Here's how the part is built. I have some questions about the finished solid (model axes, mm). Face numbers are marked on the shaded views. A direction names the side the tool comes from. Round coordinates to 2 decimals unless told otherwise and drop trailing zeros. Write each loop counter-clockwise with the first axis right and the second up, starting at its lowest first coordinate (ties: lowest second). Pieces come first, ordered by that corner, then holes. Notation, with made-up numbers: M -33,-27 L 19,-27 A12 ccw 19,-13 Z; hole C -21,-21 d11. An arc over 180 degrees is marked long. Write item = value, one per line. Start each with the question number.
(1) If we mould it in two halves opening along Y, with no side actions, what happens to the marked faces 6, 7 and 8? For each: released by +Y, released by -Y, zero draft, split by the parting line, or undercut.
(2) On a 3-axis mill with a long thin cutter (end or side, diameter ignored), from which of +Z, -Z, +X, -X, +Y, -Y can I reach the whole of each face in a straight line? I mean the marked faces 1, 2, 3, 4 and 5. Say none if no direction works.
(3) I want a section at A-A (y = 6.5). List the corners of the cut face in (x, z) for me.
(4) I want a section at C-C (y = -2.5). List the corners of the cut face in (x, z) for me, and give its area (3 significant figures).
(5) I want a section at D-D (x = 18.5). List the corners of the cut face in (y, z) for me, and give its area (3 significant figures).
(6) I want a section at B-B (z = -0.25). List the corners of the cut face in (x, y) for me, and give its area (3 significant figures).
(7) Will these pins go through, and if not, where does the flat tip stop? pin 1 Ø2 at (x, y) = (43, 12) entering from -Z; pin 2 Ø1 at (x, y) = (45.5, 10.5) entering from +Z; pin 3 Ø11 at (x, z) = (38, 1.5) entering from -Y.
(8) I need wall thicknesses on line 1 along X through (y, z) = (-0.5, 3.25); line 2 along Y through (x, z) = (6, 8.5); line 3 along X through (y, z) = (-3.25, 7.5). Which ranges of each line are inside material? Lowest first, please.
```python
from build123d import *

# Parameters (mm, degrees)
F1_DEPTH      = 5
F3_DEPTH      = 5
F3_DEPTH_BACK = 5


# Not quite as in the source:
# - a feature names something its author has since deleted; it is built from what else it names


with BuildPart() as f1:
    # F0 (on Front) → F1 (new body)
    with BuildSketch(Plane.XZ):
        Polygon((0, 9.7736853705), (0, 0), (0, -10.2263146295), (15, -10.2263146295), (15, 9.7736853705), align=None)
    extrude(amount=F1_DEPTH)

    # F2 (on Top) → F3 (join, two sides)
    with BuildSketch(Plane.XY) as f3_sk:
        Polygon((7.0152175973, 15), (7.0152175973, 0), (9.8953448171, 0), (9.8953448171, 10), (57.0152175973, 10), (57.0152175973, -4.3088319683), (60.7257795132, -4.3088319683), (60.7257795132, 15), align=None)
    extrude(amount=F3_DEPTH)
    extrude(f3_sk.sketch, amount=-F3_DEPTH_BACK)


solid = f1.part
```
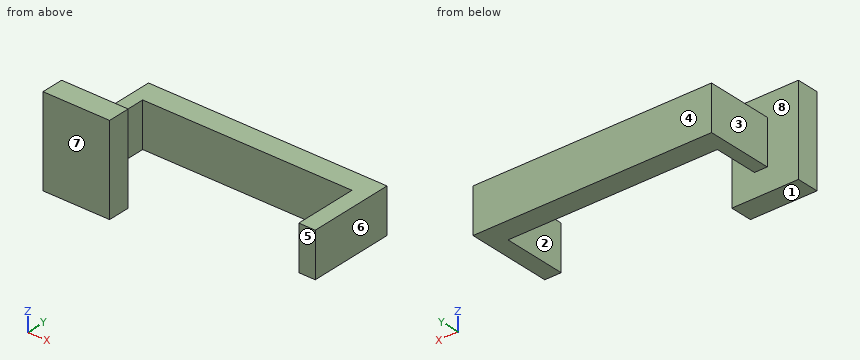
Returned:
q1.face_6 = zero draft
q1.face_7 = released by -Y
q1.face_8 = undercut
q2.face_1 = -Z, +X, -X, +Y, -Y
q2.face_2 = +Z, -Z, -Y
q2.face_3 = +Z, -Z, -X, +Y
q2.face_4 = +Z, -Z, +X, -X, +Y
q2.face_5 = +Z, -Z, +X, -Y
q3.outline = M 7.02,-5 L 9.9,-5 L 9.9,5 L 7.02,5 Z; M 57.02,-5 L 60.73,-5 L 60.73,5 L 57.02,5 Z
q4.outline = M 0,-10.23 L 15,-10.23 L 15,9.77 L 0,9.77 Z; M 57.02,-5 L 60.73,-5 L 60.73,5 L 57.02,5 Z
q4.area = 337 mm²
q5.outline = M 10,-5 L 15,-5 L 15,5 L 10,5 Z
q5.area = 50.0 mm²
q6.outline = M 0,-5 L 15,-5 L 15,0 L 9.9,0 L 9.9,10 L 57.02,10 L 57.02,-4.31 L 60.73,-4.31 L 60.73,15 L 7.02,15 L 7.02,0 L 0,0 Z
q6.area = 425 mm²
q7.pin_1 = -5
q7.pin_2 = 5
q7.pin_3 = 10
q8.line_1 = 0 to 15, 57.02 to 60.73
q8.line_2 = -5 to 0
q8.line_3 = 0 to 15
